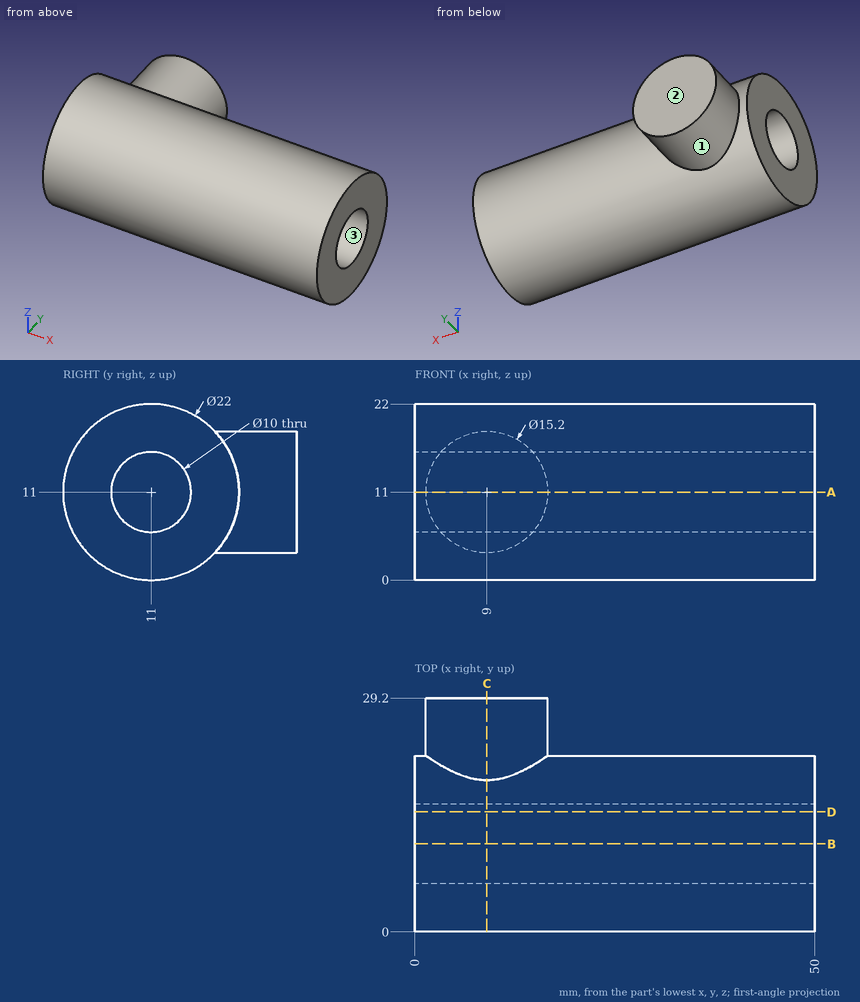
Design review of the part shown in the three views and the two pictorial views. Dimensions are in mm from the part's minimum x, y and z. Round coordinates to 2 decimals unless told otherwise and drop trailing zeros. Write each loop counter-clockwise with the first axis right and the second up, starting at its lowest first coordinate (ties: lowest second). Pieces come first, ordered by that corner, then holes.
Item 1: The part is to be moulded in two halves that separate along Z. For the marked faces 1, 2 and 3, say which applies: +Z half, -Z half, draft (parallel to the pull), parting line (faces both ways), or undercut.
Item 2: We need section D-D on y = 15. Write out the cut boundary in (x, z).
Item 3: For probe 1 along Z at (x, y) = (15, 11); probe 2 along Y at (x, z) = (32.5, 13.25); probe 3 along Z at (x, y) = (9, 10), list the stretches that pass through material, from the lowest coordinate up.
Item 4: We need section A-A on z = 11. Write out the cut boundary in (x, y).
Item 5: Clearance check with flat-ended pins moving along their axes: pin 1 Ø1 at (x, z) = (16.5, 15.5) entering from -Y; pin 2 Ø8 at (y, z) = (11, 11) entering from +X; pin 3 Ø2 at (x, y) = (27, 20) entering from -Z; pin 4 Ø5 at (x, y) = (16.5, 3.5) entering from +Z. State where each tip first meets the part, or that it passes through.
Item 6: We need section B-B on y = 11. Write out the cut boundary in (x, z), and give its area (3 significant figures).
Item 7: We need section C-C on x = 9. Write out the cut boundary in (y, z).
Returned:
1. face 1: parting line
1. face 2: draft
1. face 3: undercut
2. outline: (0, 0.75) - (50, 0.75) - (50, 8) - (0, 8) - close; (0, 14) - (50, 14) - (50, 21.25) - (0, 21.25) - close
3. probe 1: z = 0 to 6, 16 to 22
3. probe 2: y = 0.23 to 6.53, 15.47 to 21.77
3. probe 3: z = 0.05 to 6.1, 15.9 to 21.95
4. outline: (0, 0) - (50, 0) - (50, 6) - (0, 6) - close; (0, 16) - (50, 16) - (50, 22) - (16.6, 22) - (16.6, 29.2) - (1.4, 29.2) - (1.4, 22) - (0, 22) - close
5. pin 1: stops at y = 0.75
5. pin 2: passes through
5. pin 3: stops at z = 3.45
5. pin 4: stops at z = 20.8
6. outline: (0, 0) - (50, 0) - (50, 6) - (0, 6) - close; (0, 16) - (50, 16) - (50, 22) - (0, 22) - close
6. area: 600 mm2
7. outline: (18.95, 3.4) - (29.2, 3.4) - (29.2, 18.6) - (18.95, 18.6) arc R11 ccw (long way) to start; hole circle Ø10 at (11, 11)
